```python
from build123d import *

# Parameters (mm, degrees)
SKETCH1_W           = 139
SKETCH1_H           = 56
SKETCH1_R           = 1.6
SKETCH1_R_2         = 3.1
SKETCH1_R_3         = 1.5
SKETCH1_W_2         = 2.7
SKETCH1_H_2         = 1.2
BOSS_EXTRUDE1_DEPTH = 3


with BuildPart() as part:
    # Sketch1 → Boss-Extrude1 (new body)
    with BuildSketch(Plane.XY):
        with Locations((69.5, 28)):
            Rectangle(SKETCH1_W, SKETCH1_H)
        with Locations((4, 27)):
            Circle(SKETCH1_R, mode=Mode.SUBTRACT)
        with Locations((135, 27)):
            Circle(SKETCH1_R, mode=Mode.SUBTRACT)
        with Locations((135, 5)):
            Circle(SKETCH1_R, mode=Mode.SUBTRACT)
        with Locations((4, 5)):
            Circle(SKETCH1_R, mode=Mode.SUBTRACT)
        with Locations((13.518505835, 21.5)):
            Circle(SKETCH1_R, mode=Mode.SUBTRACT)
        with Locations((124, 28.19419762)):
            Circle(SKETCH1_R, mode=Mode.SUBTRACT)
        with Locations((24.645602403, 40.906620861)):
            Circle(SKETCH1_R_2, mode=Mode.SUBTRACT)
        with Locations((25.62333913, 12.743937624)):
            Circle(SKETCH1_R_2, mode=Mode.SUBTRACT)
        with Locations((111.612884483, 12.743937624)):
            Circle(SKETCH1_R_2, mode=Mode.SUBTRACT)
        with Locations((90.966366944, 35.5)):
            Circle(SKETCH1_R_2, mode=Mode.SUBTRACT)
        with Locations((74.480236578, 12.743937624)):
            Circle(SKETCH1_R_2, mode=Mode.SUBTRACT)
        with Locations((47.230023053, 12.743937624)):
            Circle(SKETCH1_R_2, mode=Mode.SUBTRACT)
        with Locations((4, 49)):
            Circle(SKETCH1_R_3, mode=Mode.SUBTRACT)
        with Locations((135, 49)):
            Circle(SKETCH1_R_3, mode=Mode.SUBTRACT)
        with Locations((24.645602403, 34.906620861)):
            Rectangle(SKETCH1_W_2, SKETCH1_H_2, mode=Mode.SUBTRACT)
        with Locations((25.62333913, 6.743937624)):
            Rectangle(SKETCH1_W_2, SKETCH1_H_2, mode=Mode.SUBTRACT)
        with Locations((111.612884483, 6.743937624)):
            Rectangle(SKETCH1_W_2, SKETCH1_H_2, mode=Mode.SUBTRACT)
        with Locations((90.966366944, 29.5)):
            Rectangle(SKETCH1_W_2, SKETCH1_H_2, mode=Mode.SUBTRACT)
        with Locations((74.480236578, 6.743937624)):
            Rectangle(SKETCH1_W_2, SKETCH1_H_2, mode=Mode.SUBTRACT)
        with Locations((47.230023053, 6.743937624)):
            Rectangle(SKETCH1_W_2, SKETCH1_H_2, mode=Mode.SUBTRACT)
    extrude(amount=BOSS_EXTRUDE1_DEPTH)


solid = part.part
```
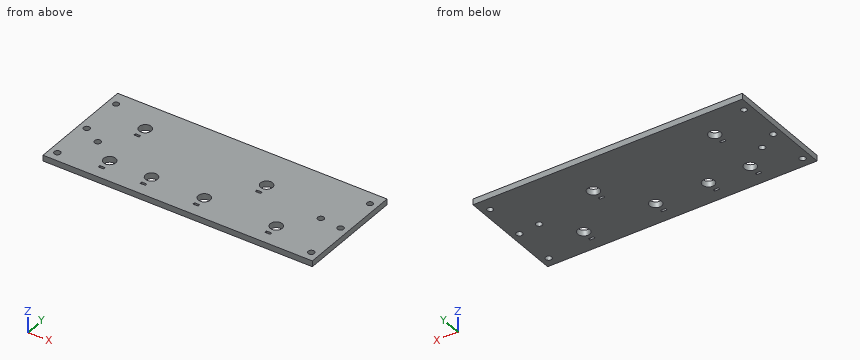
Build history of the part. All positions in model axes, mm. Round coordinates to 2 decimals unless told otherwise and drop trailing zeros. Order: outer loops, then holes, each group sorted by start corner. A loop starts at its lowest first (then second) coordinate and runs counter-clockwise, first axis right, second up. Notation, with made-up numbers: (64, -19.5) -> (111, -19.5) arc R4 cw to (111, -14.5) -> close; hole circle Ø11 at (-17, 82). An arc over 180 degrees is marked (long way). Answer in a Markdown table with one row per item.
1) Band-saw the part on C-C on y = 14. Give the cut face in (x, z), and give its area (3 significant figures).
Values:
| item | result |
|---|---|
| outline | (0, 0) -> (22.79, 0) -> (22.79, 3) -> (0, 3) -> close; (28.46, 0) -> (44.4, 0) -> (44.4, 3) -> (28.46, 3) -> close; (50.06, 0) -> (71.65, 0) -> (71.65, 3) -> (50.06, 3) -> close; (77.31, 0) -> (108.78, 0) -> (108.78, 3) -> (77.31, 3) -> close; (114.45, 0) -> (139, 0) -> (139, 3) -> (114.45, 3) -> close |
| area | 349 mm2 |
2) Band-saw the part on A-A on y = 49. Give the cut face in (x, z).
Values:
| item | result |
|---|---|
| outline | (0, 0) -> (2.5, 0) -> (2.5, 3) -> (0, 3) -> close; (5.5, 0) -> (133.5, 0) -> (133.5, 3) -> (5.5, 3) -> close; (136.5, 0) -> (139, 0) -> (139, 3) -> (136.5, 3) -> close |
3) Wall check: L1, parallel to Y at x = 75.5, z = 0.2; L2, parallel to X at y = 12, z = 1.55; L3, parallel to Y at x = 72, z = 2.35. Give the ranges that are in metal, low to high.
Values:
| item | result |
|---|---|
| L1 | 0 to 6.14, 7.34 to 9.82, 15.67 to 56 |
| L2 | 0 to 22.61, 28.63 to 44.22, 50.24 to 71.47, 77.49 to 108.6, 114.62 to 139 |
| L3 | 0 to 10.88, 14.6 to 56 |
4) Pin check, flat tip, straight feed: P1, Ø2.5, axis at x = 135, y = 49, coming from the +Z side. Stop position of the tip, or through.
Values:
| item | result |
|---|---|
| P1 | through |
5) Band-saw the part on D-D on z = 2. Give the number of separate pieces and of enclosed holes in the cut face, and give its area (3 significant figures).
Values:
| item | result |
|---|---|
| separate pieces | 1 |
| enclosed holes | 20 |
| area | 7,520 mm2 |
6) Band-saw the part on B-B on x = 135. Give the cut face in (y, z).
Values:
| item | result |
|---|---|
| outline | (0, 0) -> (3.4, 0) -> (3.4, 3) -> (0, 3) -> close; (6.6, 0) -> (25.4, 0) -> (25.4, 3) -> (6.6, 3) -> close; (28.6, 0) -> (47.5, 0) -> (47.5, 3) -> (28.6, 3) -> close; (50.5, 0) -> (56, 0) -> (56, 3) -> (50.5, 3) -> close |
